Build history of the part. All positions in model axes, mm. Coordinates: 2 decimals unless noted, no trailing zeros. Order: outer loops, then holes, each group sorted by start corner. A loop starts at its lowest first (then second) coordinate and runs counter-clockwise, first axis right, second up. Notation, with made-up numbers: (-14.75, -37) - (21.25, -37) arc R13 cw to (21.25, -28) - close; hole circle Ø2 at (17.25, 88.25). An arc over 180 degrees is marked (long way). Return JSON: item names as keys, results as strings.
from build123d import *

# Parameters (mm, degrees)
BOSS_EXTRUDE1_DEPTH = 0.5
CHAMFER3_SIZE       = 0.5
SKETCH2_R           = 1.1
CUT_EXTRUDE1_DEPTH  = 55.232831385
FILLET1_R           = 0.5
SKETCH8_W           = 2.49
SKETCH8_H           = 0.55
SKETCH8_W_2         = 2
SKETCH8_H_2         = 0.5
CUT_EXTRUDE3_DEPTH  = 0.0001
SKETCH9_W           = 2
SKETCH9_H           = 16.4
CUT_EXTRUDE4_DEPTH  = 0.0001
CHAMFER4_SIZE       = 0.3


with BuildPart() as part:
    # Sketch1 → Boss-Extrude1 (new, symmetric)
    with BuildSketch(Plane(origin=(0, 0, 0), x_dir=(1, 0, 0), z_dir=(0, 1, 0))):
        Polygon((0, 7.25), (0, -7.25), (24.45, -7.25), (24.45, -8.2), (53.6, -8.2), (53.6, 8.2), (24.45, 8.2), (24.45, 7.25), align=None)
    extrude(amount=BOSS_EXTRUDE1_DEPTH, both=True)

    # Chamfer3
    chamfer3_edges = [part.edges().sort_by_distance(p)[0] for p in [
        (53.6, 0, -8.2),
        (53.6, 0, 8.2),
    ]]
    chamfer(chamfer3_edges, length=CHAMFER3_SIZE)

    # Sketch2 → Cut-Extrude1 (cut, through all)
    with BuildSketch(Plane.XZ.offset(0.5)):
        with Locations((29.39, 8.45)):
            Circle(SKETCH2_R)
        with Locations((27.39, -8.45)):
            Circle(SKETCH2_R)
    extrude(amount=-CUT_EXTRUDE1_DEPTH, mode=Mode.SUBTRACT)

    # Fillet1
    fillet1_edges = [part.edges().sort_by_distance(p)[0] for p in [
        (24.45, 0, -8.2),
        (24.45, 0, 8.2),
    ]]
    fillet(fillet1_edges, radius=FILLET1_R)

    # Sketch8 → Cut-Extrude3 (cut)
    with BuildSketch(Plane(origin=(0, 0.5, 0), x_dir=(1, 0, 0), z_dir=(0, 1, 0))):
        with Locations((1.245, -6.975)):
            Rectangle(SKETCH8_W, SKETCH8_H)
        with Locations((1.245, 6.975)):
            Rectangle(SKETCH8_W, SKETCH8_H)
        with Locations((46.34, -7.95)):
            Rectangle(SKETCH8_W_2, SKETCH8_H_2)
        with Locations((46.34, 7.95)):
            Rectangle(SKETCH8_W_2, SKETCH8_H_2)
    extrude(amount=-CUT_EXTRUDE3_DEPTH, mode=Mode.SUBTRACT)

    # Sketch9 → Cut-Extrude4 (cut)
    with BuildSketch(Plane.XZ.offset(0.5)):
        with BuildLine():
            Line((2.09, 7.425), (0.49, 7.425))
            ThreePointArc((0.49, 7.425), (0.313223305, 7.351776695), (0.24, 7.175))
            Line((0.24, 7.175), (0.24, 6.925))
            ThreePointArc((0.24, 6.925), (0.313223305, 6.748223305), (0.49, 6.675))
            Line((0.49, 6.675), (2.09, 6.675))
            ThreePointArc((2.09, 6.675), (2.266776695, 6.748223305), (2.34, 6.925))
            Line((2.34, 6.925), (2.34, 7.175))
            ThreePointArc((2.34, 7.175), (2.266776695, 7.351776695), (2.09, 7.425))
        make_face()
        with BuildLine():
            Line((2.34, -7.175), (2.34, -6.925))
            ThreePointArc((2.34, -6.925), (2.266776695, -6.748223305), (2.09, -6.675))
            Line((2.09, -6.675), (0.49, -6.675))
            ThreePointArc((0.49, -6.675), (0.313223305, -6.748223305), (0.24, -6.925))
            Line((0.24, -6.925), (0.24, -7.175))
            ThreePointArc((0.24, -7.175), (0.313223305, -7.351776695), (0.49, -7.425))
            Line((0.49, -7.425), (2.09, -7.425))
            ThreePointArc((2.09, -7.425), (2.266776695, -7.351776695), (2.34, -7.175))
        make_face()
        with BuildLine():
            Line((26.14, -8.125), (26.14, -7.575))
            ThreePointArc((26.14, -7.575), (26.066776695, -7.398223305), (25.89, -7.325))
            Line((25.89, -7.325), (25.11, -7.325))
            ThreePointArc((25.11, -7.325), (24.933223305, -7.398223305), (24.86, -7.575))
            Line((24.86, -7.575), (24.86, -8.125))
            ThreePointArc((24.86, -8.125), (24.933223305, -8.301776695), (25.11, -8.375))
            Line((25.11, -8.375), (25.89, -8.375))
            ThreePointArc((25.89, -8.375), (26.066776695, -8.301776695), (26.14, -8.125))
        make_face()
        with Locations((46.34, 0)):
            Rectangle(SKETCH9_W, SKETCH9_H)
        with BuildLine():
            Line((25.49, 7.325), (26.89, 7.325))
            ThreePointArc((26.89, 7.325), (27.066776695, 7.398223305), (27.14, 7.575))
            Line((27.14, 7.575), (27.14, 8.125))
            ThreePointArc((27.14, 8.125), (27.066776695, 8.301776695), (26.89, 8.375))
            Line((26.89, 8.375), (25.49, 8.375))
            ThreePointArc((25.49, 8.375), (25.313223305, 8.301776695), (25.24, 8.125))
            Line((25.24, 8.125), (25.24, 7.575))
            ThreePointArc((25.24, 7.575), (25.313223305, 7.398223305), (25.49, 7.325))
        make_face()
    extrude(amount=-CUT_EXTRUDE4_DEPTH, mode=Mode.SUBTRACT)

    # Chamfer4
    chamfer4_edges = [part.edges().sort_by_distance(p)[0] for p in [
        (53.6, -0.5, 0),
        (53.6, 0.5, 0),
    ]]
    chamfer(chamfer4_edges, length=CHAMFER4_SIZE)


solid = part.part
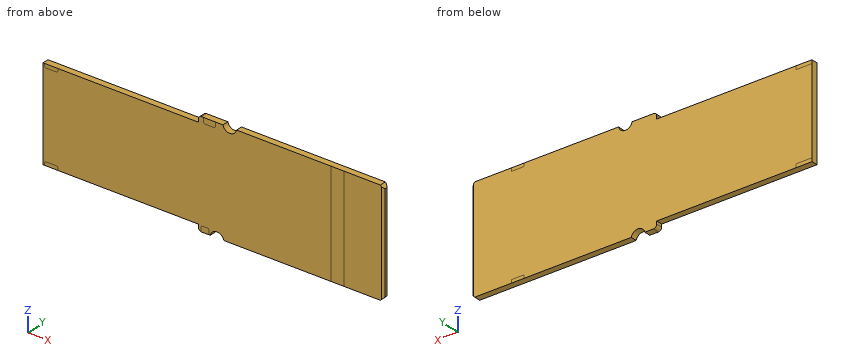
1. Cut at B-B on x = 29. Give the cut face in (y, z).
Check values:
{"outline": "(-0.5, -8.2) - (0.5, -8.2) - (0.5, 7.42) - (-0.5, 7.42) - close"}
2. Cut at A-A on x = 23. Give the cut face in (y, z).
Check values:
{"outline": "(-0.5, -7.25) - (0.5, -7.25) - (0.5, 7.25) - (-0.5, 7.25) - close"}
3. Probe L1, parallel to Z at x = 3, y = -0.3; L2, parallel to Z at x = 28, y = 0.2; L3, parallel to X at y = -0.3, z = 4. List the from-to ranges inside material, lowest first.
Check values:
{"L1": "-7.25 to 7.25", "L2": "-7.53 to 8.2", "L3": "0 to 53.5"}
